Check sheet for the modelled part. Datum: model origin and axes. Units: mm. A direction names the side the tool comes from. Give positions to 0.01 mm unless a question says otherwise; leave off trailing zeros. Write each loop counter-clockwise with the first axis right and the second up, starting at its lowest first coordinate (ties: lowest second). Pieces come first, ordered by that corner, then holes. Notation, with made-up numbers: M -25.5,44.25 L 6.5,44.25 A16 ccw 6.5,72.25 Z; hole C 28,59 d4. An arc over 180 degrees is marked long. One line per item, written item: value. Start each with the question number.
from build123d import *

# Parameters (mm, degrees)
F1_DEPTH = 723.9
F2_R     = 38.1
F3_DEPTH = 25.4


# Not quite as in the source:
# - ends of sketch curves that miss each other by under 0.0002 mm in the source are joined


with BuildPart() as f1:
    # F0 (on Front) → F1 (new body)
    with BuildSketch(Plane.XZ):
        with BuildLine():
            ThreePointArc((-8215.9952266, 774.938506), (-8224.3216631827, 771.8281073386), (-8228.56958997, 764.0204672337))
            Line((-8228.56958997, 764.0204672337), (-8323.1839632, 96.3794872))
            ThreePointArc((-8323.1839632, 96.3794872), (-8321.6915780693, 91.3252877086), (-8316.8967774, 89.138506))
            Line((-8316.8967774, 89.138506), (-8292.1428772, 89.138506))
            Line((-8292.1428772, 89.138506), (-8292.1428772, 92.313506))
            Line((-8292.1428772, 92.313506), (-8317.8109488, 92.313506))
            ThreePointArc((-8317.8109488, 92.313506), (-8319.6089965519, 93.1335462625), (-8320.1686430016, 95.0288661831))
            Line((-8320.1686430016, 95.0288661831), (-8225.4259926, 763.5749778))
            ThreePointArc((-8225.4259926, 763.5749778), (-8222.2400533643, 769.4307075881), (-8215.9952266, 771.763506))
            Line((-8215.9952266, 771.763506), (-7333.739841, 771.763506))
            ThreePointArc((-7333.739841, 771.763506), (-7327.4950142357, 769.4307075881), (-7324.3090687225, 763.5749786896))
            Line((-7324.3090687225, 763.5749786896), (-7229.6946846, 95.9339966))
            ThreePointArc((-7229.6946846, 95.9339966), (-7230.4408638812, 93.4068975271), (-7232.8382648, 92.313506))
            Line((-7232.8382648, 92.313506), (-7257.592165, 92.313506))
            Line((-7257.592165, 92.313506), (-7257.592165, 89.138506))
            Line((-7257.592165, 89.138506), (-7232.8382648, 89.138506))
            ThreePointArc((-7232.8382648, 89.138506), (-7228.0434641307, 91.3252877086), (-7226.551083115, 96.3794866168))
            Line((-7226.551083115, 96.3794866168), (-7321.1654694, 764.0204684))
            ThreePointArc((-7321.1654694, 764.0204684), (-7325.4134044173, 771.8281073386), (-7333.739841, 774.938506))
            Line((-7333.739841, 774.938506), (-8215.9952266, 774.938506))
        make_face()
    extrude(amount=F1_DEPTH)

    # F2 (on face) → F3 (cut)
    with BuildSketch(Plane.XY.offset(774.938506)):
        with Locations((-8155.8675338, -152.4)):
            Circle(F2_R)
        with Locations((-8003.4675338, -152.4)):
            Circle(F2_R)
        with Locations((-7851.0675338, -152.4)):
            Circle(F2_R)
        with Locations((-7698.6675338, -152.4)):
            Circle(F2_R)
        with Locations((-7546.2675338, -152.4)):
            Circle(F2_R)
        with Locations((-7393.8675338, -152.4)):
            Circle(F2_R)
        with Locations((-8079.6675338, -361.95)):
            Circle(F2_R)
        with Locations((-7927.2675338, -361.95)):
            Circle(F2_R)
        with Locations((-7774.8675338, -361.95)):
            Circle(F2_R)
        with Locations((-7622.4675338, -361.95)):
            Circle(F2_R)
        with Locations((-7470.0675338, -361.95)):
            Circle(F2_R)
        with Locations((-8155.8675338, -571.5)):
            Circle(F2_R)
        with Locations((-8003.4675338, -571.5)):
            Circle(F2_R)
        with Locations((-7851.0675338, -571.5)):
            Circle(F2_R)
        with Locations((-7698.6675338, -571.5)):
            Circle(F2_R)
        with Locations((-7546.2675338, -571.5)):
            Circle(F2_R)
        with Locations((-7393.8675338, -571.5)):
            Circle(F2_R)
    extrude(amount=-F3_DEPTH, mode=Mode.SUBTRACT)


solid = f1.part
1) Tool access check on faces 3 (the flat face through (-7245, -357, 92.314)), 4 (the flat face through (-8275.214, -356.883, 434.873)), 5 (the flat face through (-7781, -276, 771.764)). Record the directions out of +Z, -Z, +X, -X, +Y, -Y that give a thin tool (end or side, any length) a straight path to the whole face; none if there is none.
2) Cross-section at D-D (y = -361.95). State how many separate pieces and enclosed holes the cut face has, plus the area to 3 significant figures.
3) Draft check along Y on faces 1 (the flat face through (-8305, -357, 92.314)), 2 (the cylindrical face through (-7814.727, -140.956, 773.373)). Enter one of: released by +Y, released by -Y, zero draft, split by the parting line, or undercut.
4) Cross-section at B-B (x = -7944). Record the boundary of the cut face in (y, z), plus the area to 3 significant figures.
5) Cross-section at A-A (z = 590). Record the boundary of the cut face in (x, y), plus the area to 3 significant figures.
6) Material ranges on L1, parallel to X at y = -361, z = 773; L2, parallel to Z at x = -7881, y = -380.5; L3, parallel to X at y = -621.5, z = 530.5, recorded low to high. Write a range as from..to.
7) Gauge pin test, flat ends, axial feed: pin 1 (6 mm diameter, centred on y = -423.5, z = 648, fed in from +X); pin 2 (8 mm diameter, centred on y = -574, z = 242.5, fed in from -X); pin 3 (12 mm diameter, centred on y = -327, z = 284.5, fed in from -X). Record the tip position at first contact, or that the pin passes through.
Data:
1. face 3: +Y, -Y
1. face 4: +Z, -X, +Y, -Y
1. face 5: -Z, +Y, -Y
2. separate pieces: 6
2. enclosed holes: 0
2. area: 6,180 mm2
3. face 1: zero draft
3. face 2: undercut
4. outline: M -723.9,771.76 L -396.18,771.76 L -396.18,774.94 L -723.9,774.94 Z; M -327.72,771.76 L 0,771.76 L 0,774.94 L -327.72,774.94 Z
4. area: 2,080 mm2
5. outline: M -8253.23,-723.9 L -8250.02,-723.9 L -8250.02,0 L -8253.23,0 Z; M -7299.71,-723.9 L -7296.5,-723.9 L -7296.5,0 L -7299.71,0 Z
5. area: 4,640 mm2
6. L1: x = -8222.74..-8117.76, -8041.58..-7965.36, -7889.18..-7812.96, -7736.78..-7660.56, -7584.38..-7508.16, -7431.98..-7327
6. L2: z = 771.76..774.94
6. L3: x = -8261.66..-8258.46, -7291.28..-7288.07
7. pin 1: stops at x = -7304.3
7. pin 2: stops at x = -8303.04
7. pin 3: stops at x = -8297.37
